from build123d import *

# Parameters (mm, degrees)
PAD_DEPTH           = 5
SKETCH002_W         = 0.5
SKETCH002_H         = 2.8
POCKET_DEPTH        = 10.001
FILLET_R            = 0.5
SKETCH024_R         = 3
PAD016_DEPTH        = 5
FILLET004_R         = 1
SKETCH025_W         = 7
SKETCH025_H         = 5
PAD017_DEPTH        = 25
HOLE004_D           = 1.6
HOLE004_DEPTH       = 8
HOLE004_CBORE_D     = 3.7
HOLE004_CBORE_DEPTH = 1
HOLE004_TIPS_R      = 0.8
FILLET005_R         = 1
FILLET006_R         = 0.4
POCKET010_DEPTH     = 5.001
FILLET009_R         = 0.5


with BuildPart() as part:
    # Sketch → Pad (new body, symmetric)
    with BuildSketch(Plane.YZ):
        Polygon((-5, 7.5), (-5, 9.5), (5, 9.5), (5, 7.5), (1.55, 7.5), (1.05, 6.4), (1.55, 6.172727), (0.868182, 4.672727), (0, 5.067355), (-0.868182, 4.672727), (-1.55, 6.172727), (-1.05, 6.4), (-1.55, 7.5), align=None)
    extrude(amount=PAD_DEPTH, both=True)

    # Sketch002 → Pocket (cut, through all)
    with BuildSketch(Plane.YZ.offset(5)):
        with Locations((0, 6.1)):
            Rectangle(SKETCH002_W, SKETCH002_H)
    extrude(amount=-POCKET_DEPTH, mode=Mode.SUBTRACT)

    # Fillet
    fillet_edges = [part.edges().sort_by_distance(p)[0] for p in [
        (0, 0.868182, 4.672727),
        (0, -0.868182, 4.672727),
    ]]
    fillet(fillet_edges, radius=FILLET_R)

    # Sketch024 (on Face2 of Pad) → Pad016 (join)
    with BuildSketch(Plane(origin=(0, 0, 9.5), x_dir=(0, -1, 0), z_dir=(0, 0, 1))):
        Circle(SKETCH024_R)
    extrude(amount=PAD016_DEPTH)

    # Fillet004
    fillet004_edges = [part.edges().sort_by_distance(p)[0] for p in [
        (0, 3, 9.5),
    ]]
    fillet(fillet004_edges, radius=FILLET004_R)

    # Sketch025 (on DatumPlane) → Pad017 (join)
    with BuildSketch(Plane(origin=(0, -5, 0), x_dir=(0, 0, -1), z_dir=(0, -1, 0))):
        with Locations((-11, 2.5)):
            Rectangle(SKETCH025_W, SKETCH025_H)
    extrude(amount=-PAD017_DEPTH)

    # Hole004
    with Locations(Plane(origin=(0, 0, 14.5), x_dir=(0, -1, 0), z_dir=(0, 0, 1))):
        with Locations((0, 0)):
            CounterBoreHole(HOLE004_D / 2, HOLE004_CBORE_D / 2, HOLE004_CBORE_DEPTH, depth=HOLE004_DEPTH)

    # Hole004 tips → Hole004 tip 1 section 0
    with BuildSketch(Plane(origin=(0, 0, 6.5), x_dir=(0, -1, 0), z_dir=(0, 0, 1)), mode=Mode.PRIVATE) as hole004_tip_1_s0:
        Circle(HOLE004_TIPS_R)
    loft([hole004_tip_1_s0.sketch, Vertex(0, 0, 6.019312)], mode=Mode.SUBTRACT)

    # Fillet005
    fillet005_edges = [part.edges().sort_by_distance(p)[0] for p in [
        (0, -5, 12),
        (0, -4, 14.5),
        (0, 11.5, 14.5),
        (0, 20, 11),
        (2.5, 20, 7.5),
        (0, 12.5, 7.5),
        (2.5, -5, 14.5),
        (2.5, 20, 14.5),
    ]]
    fillet(fillet005_edges, radius=FILLET005_R)

    # Fillet006
    fillet006_edges = [part.edges().sort_by_distance(p)[0] for p in [
        (-2.5, -5, 9.5),
        (-5, 0, 9.5),
        (-2.5, 5, 9.5),
        (0.5, -5, 9.5),
        (-5, 5, 8.5),
        (-5, -5, 8.5),
        (5, 7.5, 14.5),
        (5, 19.707107, 14.207107),
        (5, 20, 11),
        (5, 19.707107, 7.792893),
        (5, 10.275, 7.5),
        (5, -5, 10.5),
        (5, -4.707107, 14.207107),
        (5, -3.275, 7.5),
        (-2.5, 5, 7.5),
        (0.5, 5, 7.5),
        (-5, 3.275, 7.5),
        (-5, -3.275, 7.5),
        (0, -5, 7.5),
    ]]
    fillet(fillet006_edges, radius=FILLET006_R)

    # Sketch027 (on DatumPlane) → Pocket010 (cut, through all)
    with BuildSketch(Plane(origin=(0, 0, 0), x_dir=(0, 1, 0), z_dir=(-1, 0, 0))):
        with BuildLine():
            Line((7, -9.4), (16.5, -9.4))
            ThreePointArc((16.5, -12.6), (18.1, -11), (16.5, -9.4))
            Line((16.5, -12.6), (7, -12.6))
            ThreePointArc((7, -9.4), (5.4, -11), (7, -12.6))
        make_face()
    extrude(amount=-POCKET010_DEPTH, mode=Mode.SUBTRACT)

    # Fillet009
    fillet009_edges = [part.edges().sort_by_distance(p)[0] for p in [
        (0, 11.75, 12.6),
        (0, 18.1, 11),
        (0, 11.75, 9.4),
        (0, 5.4, 11),
    ]]
    fillet(fillet009_edges, radius=FILLET009_R)


with BuildPart() as part_1:
    # Body001 placement: moved
    add(part.part.moved(Location((-37.45, 0, 0))))


solid = part_1.part
The model under review builds one solid part; all positions refer to its coordinate system, in mm. A direction names the side the tool comes from. Give positions to 0.01 mm unless a question says otherwise; leave off trailing zeros. Order: outer loops, then holes, each group sorted by start corner. A loop starts at its lowest first (then second) coordinate and runs counter-clockwise, first axis right, second up. Notation, with made-up numbers: (-36, 13.25) -> (-17, 13.25) arc R21 cw to (-17, 27.25) -> close; hole circle Ø2 at (-10.75, 60.25). An arc over 180 degrees is marked (long way). Write item = value, one per line. Start each with the question number.
(1) Take a section at C-C (y = 0). Write out the cut boundary in (x, z).
(2) For L1, parallel to Z at x = -35, y = 7.5; L2, parallel to Z at x = -33, y = 2; L3, parallel to Y at x = -40.25, z = 8.75, list the stretches that pass through material, from the lowest coordinate up. Write a range as from..to.
(3) For pin 1 Ø3 at (x, z) = (-38.5, 10) entering from +Y; pin 2 Ø1.1 at (x, y) = (-38, 0) entering from +Z; pin 3 Ø2.5 at (y, z) = (13.5, 10.5) entering from -X, all flat-tipped, find the tip position at first contact; note any pin that passes through.
(4) Take a section at A-A (z = 11). Write out the cut boundary in (x, y), plus the area to 3 significant figures.
(5) Take a section at B-B (x = -35). Write out the cut boundary in (y, z), plus the area to 3 significant figures.
(6) Take a section at D-D (z = 12.25). State how many separate pieces and enclosed holes the cut face has, plus the area to 3 significant figures.
(7) Tool access review of faces 1 (the flat face through (-35, 12, 9.4)), 2 (the cylindrical face through (-37.165, -4.699, 11.269)), 3 (the flat face through (-37, -3, 7.5)): name each direction out of +Z, -Z, +X, -X, +Y, -Y from which nothing blocks a thin tool from reaching the whole face with its end or side.
(8) Draft analysis for pull direction Y (two halves, no side actions). For faces 4 (the flat face through (-37.38, -1.31, 5.64)), 5 (the cylindrical face through (-34.7, 18.1, 11)), 6 (the flat face through (-35, 8, 7.5)), state which applies: +Y half, -Y half, draft (parallel to the pull), parting line (faces both ways), or undercut.
Returned:
q1.outline = (-42.45, 7.5) -> (-38.25, 7.5) -> (-38.25, 13.5) -> (-39.3, 13.5) -> (-39.3, 14.5) -> (-40.45, 14.5) -> (-40.45, 10.5) arc R1 cw to (-41.45, 9.5) -> (-42.05, 9.5) arc R0.4 ccw to (-42.45, 9.1) -> close; (-36.65, 7.5) -> (-32.45, 7.5) -> (-32.45, 14.1) arc R0.4 ccw to (-32.85, 14.5) -> (-35.6, 14.5) -> (-35.6, 13.5) -> (-36.65, 13.5) -> close
q2.L1 = 7.5..9.4, 12.6..14.5
q2.L2 = 7.5..14.5
q2.L3 = -5..5
q3.pin_1 = 19.84
q3.pin_2 = 13.5
q3.pin_3 = -37.31
q4.outline = (-37.45, -4) arc R1 ccw to (-36.45, -5) -> (-32.85, -5) arc R0.4 ccw to (-32.45, -4.6) -> (-32.45, 5.4) -> (-36.95, 5.4) arc R0.5 ccw to (-37.45, 4.9) -> (-37.45, 3) arc R3 ccw to (-37.45, -3) -> close; (-37.45, 18.6) arc R0.5 ccw to (-36.95, 18.1) -> (-32.45, 18.1) -> (-32.45, 19.6) arc R0.4 ccw to (-32.85, 20) -> (-36.45, 20) arc R1 ccw to (-37.45, 19) -> close; hole circle Ø1.6 at (-37.45, 0)
q4.area = 73.0 mm²
q5.outline = (-5, 7.9) arc R0.4 ccw to (-4.6, 7.5) -> (-1.55, 7.5) -> (-1.05, 6.4) -> (-1.55, 6.17) -> (-1.08, 5.13) arc R0.5 ccw to (-0.41, 4.88) -> (-0.25, 4.95) -> (-0.25, 7.5) -> (0.25, 7.5) -> (0.25, 4.95) -> (0.41, 4.88) arc R0.5 ccw to (1.08, 5.13) -> (1.55, 6.17) -> (1.05, 6.4) -> (1.55, 7.5) -> (19, 7.5) arc R1 ccw to (20, 8.5) -> (20, 13.5) arc R1 ccw to (19, 14.5) -> (-4, 14.5) arc R1 ccw to (-5, 13.5) -> close; hole (7, 9.4) -> (16.5, 9.4) arc R1.6 ccw to (16.5, 12.6) -> (7, 12.6) arc R1.6 ccw to start
q5.area = 141 mm²
q6.separate_pieces = 2
q6.enclosed_holes = 1
q6.area = 79.0 mm²
q7.face_1 = +X, -X
q7.face_2 = +Z, -X, -Y
q7.face_3 = -Z, +X, -X, -Y
q8.face_4 = -Y half
q8.face_5 = undercut
q8.face_6 = draft
